Verification items for the finished model (mm, model axes). A direction names the side the tool comes from. Give positions to 0.01 mm unless a question says otherwise; leave off trailing zeros. Loops run counter-clockwise (first coordinate to the right, second up) from the corner with the lowest first, then second, coordinate; pieces in that order, holes last. Notation, with made-up numbers: M -2,23.25 L 6,23.25 A26 cw 6,59.25 Z; hole C 75.5,32 d11. An arc over 180 degrees is marked long. Put each result on its own line as item: value. Start each with the question number.
Autodesk Inventor part; units mm, degrees
ref_plane "YZ Plane" through (0, 0, 0) normal (1, 0, 0) x (0, 1, 0)
ref_plane "XZ Plane" through (0, 0, 0) normal (0, 1, 0) x (-1, 0, 0)
ref_plane "XY Plane" through (0, 0, 0) normal (0, 0, 1) x (1, 0, 0)
ref_plane "Work Plane1" through (0, 0, 0) normal (0, 0, 1) x (1, 0, 0)
ref_plane "Work Plane2" through (13.4154, -42.9082, 9) normal (0, 0, -1) x (-0.9086751, -0.417504, 0)
sketch "Sketch1" plane through (13.4154, -42.9082, 9) normal (0, 0, -1) x (-0.9086751, -0.417504, 0)
  line L0 (20.066, 26.9166) -> (20.066, 62.7742)
  line L1 (20.066, 62.7742) -> (17.9288, 64.9114)
  line L2 (17.9288, 64.9114) -> (-17.9288, 64.9114)
  line L3 (-17.9288, 64.9114) -> (-20.066, 62.7742)
  line L4 (-20.066, 62.7742) -> (-20.066, 26.9166)
  line L5 (-20.066, 26.9166) -> (-17.9288, 24.7794)
  line L6 (-17.9288, 24.7794) -> (17.9288, 24.7794)
  line L7 (17.9288, 24.7794) -> (20.066, 26.9166)
  circle A0 centre (-15, 59.8454) radius 3.2639
  circle A1 centre (15, 59.8454) radius 3.2639
  circle A2 centre (-15, 29.8455) radius 3.2639
  circle A3 centre (15, 29.8455) radius 3.2639
  circle A4 centre (0, 44.8454) radius 13.3985
  line L8 (8, 50.8454) -> (-7.5, 50.8454) construction
  line L9 (-7.5, 50.8454) -> (-7.5, 37.3454) construction
  line L10 (-7.5, 37.3454) -> (8, 37.3454) construction
  line L11 (8, 37.3454) -> (8, 50.8454) construction
  circle A5 centre (-17.5, 54.8454) radius 1 construction
  circle A6 centre (-11, 34.3454) radius 1 construction
  circle A7 centre (10.5, 49.8454) radius 1 construction
  arc A8 (-15.8555, 56.5454) -> (-16.8555, 57.5454) centre (-16.8555, 56.5454) ccw construction
  line L12 (-15.8555, 56.5454) -> (-15.8555, 53.8078) construction
  arc A9 (-15.8555, 53.8078) -> (-14.8555, 52.8078) centre (-14.8555, 53.8078) ccw construction
  line L13 (-14.8555, 52.8078) -> (12, 52.8078) construction
  arc A10 (13, 51.8078) -> (12, 52.8078) centre (12, 51.8078) ccw construction
  line L14 (13, 51.8078) -> (13, 49.2425) construction
  arc A11 (12, 48.2425) -> (13, 49.2425) centre (12, 49.2425) ccw construction
  line L15 (12, 48.2425) -> (11, 48.2425) construction
  arc A12 (11, 48.2425) -> (10, 47.2425) centre (11, 47.2425) ccw construction
  line L16 (10, 47.2425) -> (10, 35.7078) construction
  line L17 (10, 35.7078) -> (-8.4723, 35.7078) construction
  arc A13 (-8.4723, 35.7078) -> (-9.4723, 34.7078) centre (-8.4723, 34.7078) ccw construction
  line L18 (-9.4723, 34.7078) -> (-9.4723, 32.8454) construction
  arc A14 (-10.4723, 31.8454) -> (-9.4723, 32.8454) centre (-10.4723, 32.8454) ccw construction
  line L19 (-10.4723, 31.8454) -> (-20, 31.8454) construction
  line L20 (-20, 31.8454) -> (-20, 57.5454) construction
  line L21 (-20, 57.5454) -> (-16.8555, 57.5454) construction
  line L22 (8, 37.3454) -> (-7.5, 37.3454)
  line L23 (-7.5, 37.3454) -> (-7.5, 50.8454)
  line L24 (-7.5, 50.8454) -> (8, 50.8454)
  line L25 (8, 50.8454) -> (8, 37.3454)
  circle A15 centre (10.5, 49.8454) radius 1
  circle A16 centre (-17.5, 54.8454) radius 1
  circle A17 centre (-11, 34.3454) radius 1
  circle A18 centre (15, 29.8455) radius 3.05
  circle A19 centre (-15, 29.8455) radius 3.05
  circle A20 centre (-15, 59.8454) radius 3.05
  circle A21 centre (15, 59.8454) radius 3.05
  point P0 (-5.7241, 44.5906)
  dimension "d2" = 6.1
  dimension "d3" = 6.1
  dimension "d4" = 6.1
  dimension "d5" = 6.1
extrude "Extrusion1" add sketch "Sketch1" along normal blind 8 contours L7 L6 L5 L4 L3 L2 L1 L0 | A0 | A1 | A2 | A3 | A4
shell "Shell1" thickness 2 removed faces 1 at (-8.0461, 9.7896, 1)
properties part number "10_Adapter_KES400_Thorlabs"
Q1. Cross-section at B-B, the plane z = 8. State how many separate pieces and enclosed holes the cut face has, then the cut area to 3 significant figures.
Q2. Set-up check for faces 4 (the face through (3.26, 1.95, 4.04)), 5 (the face through (1.86, 0.21, 5.06)), 6 (the face through (-14.62, -27.36, 5.06)): record each of +Z, -Z, +X, -X, +Y, -Y from which the full face is reachable in a straight line by a thin tool's end or side.
Q3. Go/stop test with flat-tipped pins: pin 1 (2 mm diameter, centred on x = 11, z = 8, fed in from +Y); pin 2 (4 mm diameter, centred on x = 9.5, z = 3.5, fed in from -Y); pin 3 (1 mm diameter, centred on y = 6.5, z = 6, fed in from -X). Record where each tip stops, or that it passes through.
Q4. Cross-section at C-C, the plane y = -21. Record the boundary of the cut face in (x, z), then the cut area to 3 significant figures.
Q5. Scan lines: L1, parallel to Y at x = 12, z = 5; L2, parallel to X at y = -13, z = 3; L3, parallel to X at y = 17, z = 2.5. Record each from-to range of solid material in increasing order.
Q6. Release check for a two-part mould opening along Y. For faces 1 (the face through (-13.91, 15.97, 5.06)), 2 (the face through (3, 2, 1)), 3 (the face through (-12.99, 14.194, 4.042)) record: pulls with the +Y half, pulls with the -Y half, needs draft (parallel to the pull), parting line crosses it, or undercut.
Q7. Cross-section at A-A, the plane x = -27. Record the boundary of the cut face in (y, z).
Ans:
1. separate pieces: 1
1. enclosed holes: 8
1. area: 1,270 mm^2
2. face 4: -Z
2. face 5: +Z, -Z
2. face 6: +Z, -Z, -X, -Y
3. pin 1: stops at y = 12.59
3. pin 2: stops at y = -18.36
3. pin 3: stops at x = -30.94
4. outline: M -18.73,1 L -15.54,1 L -15.54,9 L -18.73,9 Z; M -9.81,1 L -7.74,1 L -7.74,7 L -3.04,7 L -3.04,1 L 1.75,1 L 1.75,9 L -9.81,9 Z
4. area: 89.9 mm^2
5. L1: y = -16.29 to -14.09, -13.86 to -11.14, -7.91 to -5.19, 3.44 to 8.23
5. L2: x = -22.41 to -20.21, -11.33 to -6.15, 10.92 to 19.16
5. L3: x = -11.67 to -6.88, -2.94 to -0.9, 5.02 to 7.97
6. face 1: pulls with the +Y half
6. face 2: needs draft
6. face 3: undercut
7. outline: M -3.01,1 L 2.75,1 L 2.75,9 L -3.01,9 Z; M 7.67,1 L 9.96,1 L 9.96,9 L 7.67,9 Z
